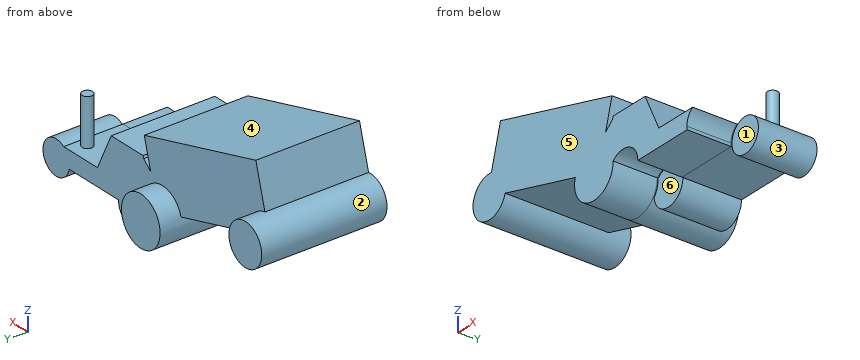
from build123d import *

# Parameters (mm, degrees)
F1_DEPTH  = 114.3
F2_R      = 14.7641240752
F3_DEPTH  = 132.08
F5_DEPTH  = 165.1
F6_DEPTH  = 53.34
F7_W      = 167.64
F7_H      = 75.5490642041
F8_DEPTH  = 416.56
F9_DEPTH  = 104.14
F10_R     = 58.9096936167
F10_R_2   = 69.3638510651
F11_DEPTH = 228.6
F12_DEPTH = 124.46


with BuildPart() as f1:
    # F0 (on Front) → F1 (new body)
    with BuildSketch(Plane.XZ):
        Polygon((-152.2679626942, 91.6335880756), (-174.4953691959, 12.3544447124), (-143.3922946453, 68.4929564595), (-127.1618189825, 113.5505846584), align=None)
        Polygon((-143.3922946453, 68.4929564595), (-174.4953691959, 12.3544447124), (-88.5811317712, -30.8491028845), (-88.5811317712, 68.4929564595), align=None)
        Polygon((-127.1618189825, 113.5505846584), (-143.3922946453, 68.4929564595), (-88.5811317712, 68.4929564595), (-33.7699688971, 68.4929564595), (-10.2984756231, 120.4584985971), (-119.2487329245, 120.4584985971), align=None)
        Polygon((-88.5811317712, 68.4929564595), (-88.5811317712, -30.8491028845), (29.068255797, -30.8491028845), (8.9511722326, 17.8852565587), (-33.7699688971, 68.4929564595), align=None)
        Polygon((-124.6734783053, 120.4584985971), (-127.1618189825, 113.5505846584), (-119.2487329245, 120.4584985971), align=None)
        Polygon((8.9511722326, 17.8852565587), (29.068255797, -30.8491028845), (200.966194272, -30.8491028845), (200.966194272, 17.8852565587), (131.0636848211, 17.8852565587), (39.2291881144, 17.8852565587), align=None)
        Polygon((-10.2984756231, 120.4584985971), (-33.7699688971, 68.4929564595), (8.9511722326, 17.8852565587), (39.2291881144, 17.8852565587), align=None)
    extrude(amount=F1_DEPTH)

    # F2 (on face) → F3 (join)
    with BuildSketch(Plane.XY.offset(17.8852565587)):
        with Locations((132.660344243, -44.7543635964)):
            Circle(F2_R)
    extrude(amount=F3_DEPTH)

    # F4 (on face) → F5 (join)
    with BuildSketch(Plane(origin=(0, 0, 0), x_dir=(-1, 0, 0), z_dir=(0, 1, 0))):
        with BuildLine():
            ThreePointArc((140.7021095386, -30.8491028845), (88.5811317712, 21.2718748828), (36.4601540038, -30.8491028845))
            ThreePointArc((36.4601540038, -30.8491028845), (88.5811317712, -82.9700806519), (140.7021095386, -30.8491028845))
        make_face()
        with BuildLine():
            ThreePointArc((-139.8416826612, -21.4376766235), (-234.8171624105, -16.7085714313), (-140.7812567162, -30.8491028845))
            ThreePointArc((-140.7812567162, -30.8491028845), (-140.0771585543, -26.1667818156), (-139.8416826612, -21.4376766235))
        make_face()
    extrude(amount=-F5_DEPTH)

    # F6 (add): a face of the model
    f6_faces = [f1.faces().sort_by_distance(p)[0] for p in [
        (-32.0897758633, -114.3, 39.2066158894),
    ]]
    extrude(f6_faces, amount=F6_DEPTH)

    # F7 (on face) → F8 (join)
    with BuildSketch(Plane(origin=(-164.9898592959, 0, 46.2580259532), x_dir=(0, -1, 0), z_dir=(-0.9628717361, 0, 0.2699592929))):
        with Locations((83.82, -9.3836272135)):
            Rectangle(F7_W, F7_H)
    extrude(amount=F8_DEPTH)

    # F9 (add): a face of the model
    f9_faces = [f1.faces().sort_by_distance(p)[0] for p in [
        (-357.8723958787, -83.82, 129.8219473654),
    ]]
    extrude(f9_faces, amount=F9_DEPTH)

    # F10 (on face) → F11 (join)
    with BuildSketch(Plane.XZ.offset(167.64)):
        with Locations((-570.314151911, 110.9217789702)):
            Circle(F10_R)
        with Locations((-194.5015435206, 5.555610003)):
            Circle(F10_R_2)
    extrude(amount=-F11_DEPTH)

    # F12 (add): a face of the model
    f12_faces = [f1.faces().sort_by_distance(p)[0] for p in [
        (-283.3393159962, -167.64, 105.4244484486),
    ]]
    extrude(f12_faces, amount=F12_DEPTH)


solid = f1.part
Model file for the job. Use its own axes, mm. Face numbers are marked on the shaded views. A direction names the side the tool comes from. Coordinates: 2 decimals unless noted, no trailing zeros. Write each loop counter-clockwise with the first axis right and the second up, starting at its lowest first coordinate (ties: lowest second). Pieces come first, ordered by that corner, then holes. Notation, with made-up numbers: (-18, -30) - (27, -30) arc R19 ccw to (27, 4) - close; hole circle Ø8 at (50, 76). An arc over 180 degrees is marked (long way). Write each question's results on one line, items separated by ' | '. Start each with the question number.
1) Cut at A-A (y = -227.5). Write the cut outline in (x, z), then the cut area to 3 significant figures.
2) Cut at B-B (x = -164). Write the cut outline in (y, z), then the cut area to 3 significant figures.
3) Probe line 1 along X through (y, z) = (-109, -41); line 2 along Y through (x, z) = (-221, 172.5); line 3 along Z through (x, y) = (-88, -85). List the from-to ranges inside material, lowest first. Write a range as from..to.
4) Mould opens along X. For the marked faces 1, 2, 3 and 4 say: pulls with the +X half, pulls with the -X half, needs draft (parallel to the pull), parting line crosses it, or undercut.
5) 3-axis set-ups, long thin cutter, end or side, ignore diameter. For the marked faces 5 and 6: which of +Z, -Z, +X, -X, +Y, -Y reach the whole face in a straight line?
6) Cut at D-D (z = 209). Write the cut outline in (x, y), then the cut area to 3 significant figures.
7) Cut at C-C (y = 26). Write the cut outline in (x, z).
8) Flat gauge pins, fed straight in: P1, Ø3, axis at x = -24.5, y = -161, coming from the -Z side; P2, Ø2, axis at y = -57, z = 192, coming from the -X side; P3, Ø15, axis at x = 132.5, y = -47.5, coming from the +Z side. Where does each tip first touch, or does it go through?
Returned:
1) outline: (-563.09, 169.39) arc R58.91 ccw (long way) to (-513.59, 95.02) - (-261.29, 24.28) arc R69.36 ccw (long way) to (-125.14, 6.3) arc R52.12 cw to (-36.46, -30.85) - (140.78, -30.85) arc R47.61 cw to (160.61, 17.89) - (39.23, 17.89) - (-10.3, 120.46) - (-124.67, 120.46) - (-127.16, 113.55) - (-152.27, 91.63) - (-129.21, 173.87) - (-530.31, 286.32) - close | area: 118,000 mm^2
2) outline: (-292.1, -56.74) - (60.96, -56.74) - (60.96, 67.85) - (0, 67.85) - (0, 183.62) - (-292.1, 183.62) - close | area: 77,800 mm^2
3) line 1: -245.92..-143.08, -139.7..-37.46, 144.05..230.85 | line 2: -292.1..0 | line 3: -82.97..120.46
4) face 1: needs draft | face 2: undercut | face 3: undercut | face 4: pulls with the +X half
5) face 5: +Z, -Z, +X, -X, -Y | face 6: -Z, -Y
6) outline: (-551.98, -292.1) - (-254.52, -292.1) - (-254.52, 0) - (-551.98, 0) - close | area: 86,900 mm^2
7) outline: circle Ø117.82 at (-570.31, 110.92); circle Ø138.73 at (-194.5, 5.56)
8) P1: z = -30.85 | P2: x = -557.03 | P3: z = 149.97
